Autodesk Inventor part; units mm, degrees
ref_plane "YZ Plane" through (0, 0, 0) normal (1, 0, 0) x (0, 1, 0)
ref_plane "XZ Plane" through (0, 0, 0) normal (0, 1, 0) x (-1, 0, 0)
ref_plane "XY Plane" through (0, 0, 0) normal (0, 0, 1) x (1, 0, 0)
sketch "Sketch1" plane through (0, 0, 0) normal (0, 1, 0) x (-1, 0, 0)
  circle A0 centre (0, 0) radius 8.75
  circle A1 centre (0, 0) radius 1.5
  line L0 (0, 0) -> (6.35, 0)
  circle A2 centre (6.35, 0) radius 1.1
  circle A3 centre (0, 6.35) radius 1.1
  circle A4 centre (-6.35, 0) radius 1.1
  circle A5 centre (0, -6.35) radius 1.1
  dimension "d0" = 17.5
  dimension "d1" = 3
  dimension "d2" = 6.35
  dimension "d3" = 2.2
  dimension "d6" = 360
extrude "Extrusion1" add sketch "Sketch1" along normal blind 5
properties part number "Hub"
CAD build for the part. Positions are in the model's coordinates, mm. Give positions to 0.01 mm unless a question says otherwise; leave off trailing zeros. Write each loop counter-clockwise with the first axis right and the second up, starting at its lowest first coordinate (ties: lowest second). Pieces come first, ordered by that corner, then holes. Notation, with made-up numbers: M 78,54.25 L 111,54.25 A21 ccw 111,87.25 Z; hole C 19.25,54 d10. An arc over 180 degrees is marked long. Return JSON: item names as keys, results as strings. Group by question number.
(1) Drill centre lines: L1, parallel to Z at x = 0, y = 3.75; L2, parallel to Z at x = 6.35, y = 3.25; L3, parallel to X at y = 0.55, z = -7.25. Where is each one in solid material? Low to high. Write a range as [from, to].
(2) Band-saw the part on B-B (y = 3.75). Give the cut face in (x, z), and give its area (3 significant figures).
(3) Band-saw the part on D-D (x = -7). Give the cut face in (y, z).
(4) Flat gauge pins, fed straight in: pin 1 Ø3.5 at (x, z) = (-6.35, 0) entering from -Y; pin 2 Ø1.5 at (y, z) = (2, -2.5) entering from +X. Where does each tip first touch, or does it go through?
(5) Band-saw the part on A-A (z = 0). Give the cut face in (x, y), and give its area (3 significant figures).
(6) Band-saw the part on C-C (z = 6.35). Give the cut face in (x, y).
Entries:
{
 "1": {"L1": "z = [-8.75, -7.45], [-5.25, -1.5], [1.5, 5.25], [7.45, 8.75]", "L2": "z = [-6.02, -1.1], [1.1, 6.02]", "L3": "x = [-4.9, -0.63], [0.63, 4.9]"},
 "2": {"outline": "C 0,0 d17.5; hole C -6.35,0 d2.2; hole C 0,0 d3; hole C 0,-6.35 d2.2; hole C 0,6.35 d2.2; hole C 6.35,0 d2.2", "area": "218 mm^2"},
 "3": {"outline": "M 0,-5.25 L 5,-5.25 L 5,-0.89 L 0,-0.89 Z; M 0,0.89 L 5,0.89 L 5,5.25 L 0,5.25 Z"},
 "4": {"pin 1": "stops at y = 0", "pin 2": "stops at x = 8.57"},
 "5": {"outline": "M -8.75,0 L -7.45,0 L -7.45,5 L -8.75,5 Z; M -5.25,0 L -1.5,0 L -1.5,5 L -5.25,5 Z; M 1.5,0 L 5.25,0 L 5.25,5 L 1.5,5 Z; M 7.45,0 L 8.75,0 L 8.75,5 L 7.45,5 Z", "area": "50.5 mm^2"},
 "6": {"outline": "M -6.02,0 L -1.1,0 L -1.1,5 L -6.02,5 Z; M 1.1,0 L 6.02,0 L 6.02,5 L 1.1,5 Z"}
}
